from build123d import *

# Parameters (mm, degrees)
F0_W     = 10
F0_H     = 10
F1_DEPTH = 3.75


with BuildPart() as f1:
    # F0 (on Front) → F1 (new body, symmetric)
    with BuildSketch(Plane.XZ):
        with BuildLine():
            Line((13.240477, 26.920062), (-1.299121, 22.463483))
            Line((-1.299121, 22.463483), (0.005236, 30))
            ThreePointArc((0.005236, 30), (-0.994655, 29.983506), (-1.993441, 29.933697))
            Line((-1.993441, 29.933697), (-12.356813, 18.804386))
            Line((-12.356813, 18.804386), (-14.995465, 25.98338))
            ThreePointArc((-14.995465, 25.98338), (-15.85315, 25.469151), (-16.693219, 24.926621))
            Line((-16.693219, 24.926621), (-20.103507, 10.10667))
            Line((-20.103507, 10.10667), (-25.978144, 15.004534))
            ThreePointArc((-25.978144, 15.004534), (-26.463806, 14.130356), (-26.920062, 13.240477))
            Line((-26.920062, 13.240477), (-22.463483, -1.299121))
            Line((-22.463483, -1.299121), (-30, 0.005236))
            ThreePointArc((-30, 0.005236), (-29.983506, -0.994655), (-29.933697, -1.993441))
            Line((-29.933697, -1.993441), (-18.804386, -12.356813))
            Line((-18.804386, -12.356813), (-25.98338, -14.995465))
            ThreePointArc((-25.98338, -14.995465), (-25.469151, -15.85315), (-24.926621, -16.693219))
            Line((-24.926621, -16.693219), (-10.10667, -20.103507))
            Line((-10.10667, -20.103507), (-15.004534, -25.978144))
            ThreePointArc((-15.004534, -25.978144), (-14.130356, -26.463806), (-13.240477, -26.920062))
            Line((-13.240477, -26.920062), (1.299121, -22.463483))
            Line((1.299121, -22.463483), (-0.005236, -30))
            ThreePointArc((-0.005236, -30), (0.994655, -29.983506), (1.993441, -29.933697))
            Line((1.993441, -29.933697), (12.356813, -18.804386))
            Line((12.356813, -18.804386), (14.995465, -25.98338))
            ThreePointArc((14.995465, -25.98338), (15.85315, -25.469151), (16.693219, -24.926621))
            Line((16.693219, -24.926621), (20.103507, -10.10667))
            Line((20.103507, -10.10667), (25.978144, -15.004534))
            ThreePointArc((25.978144, -15.004534), (26.463806, -14.130356), (26.920062, -13.240477))
            Line((26.920062, -13.240477), (22.463483, 1.299121))
            Line((22.463483, 1.299121), (30, -0.005236))
            ThreePointArc((30, -0.005236), (29.983506, 0.994655), (29.933697, 1.993441))
            Line((29.933697, 1.993441), (18.804386, 12.356813))
            Line((18.804386, 12.356813), (25.98338, 14.995465))
            ThreePointArc((25.98338, 14.995465), (25.469151, 15.85315), (24.926621, 16.693219))
            Line((24.926621, 16.693219), (10.10667, 20.103507))
            Line((10.10667, 20.103507), (15.004534, 25.978144))
            ThreePointArc((15.004534, 25.978144), (14.130356, 26.463806), (13.240477, 26.920062))
        make_face()
        Rectangle(F0_W, F0_H, mode=Mode.SUBTRACT)
    extrude(amount=F1_DEPTH, both=True)


solid = f1.part
Part model, mm, in its own coordinate system. A direction names the side the tool comes from. Coordinates: 2 decimals unless noted, no trailing zeros. Order: outer loops, then holes, each group sorted by start corner. A loop starts at its lowest first (then second) coordinate and runs counter-clockwise, first axis right, second up.
(1) Slice it at D-D, the plane x = -9. Write the cut outline in (y, z).
Check sheet entries:
outline: (-3.75, -25.62) - (3.75, -25.62) - (3.75, 22.41) - (-3.75, 22.41) - close
(2) Slice it at A-A, the plane z = -4. Write the cut outline in (x, y).
Check sheet entries:
outline: (-27.78, -3.75) - (-5, -3.75) - (-5, 3.75) - (-27.78, 3.75) - close; (5, -3.75) - (24.09, -3.75) - (24.09, 3.75) - (5, 3.75) - close
(3) Pin check, flat tips, straight feed: pin 1 Ø4 at (x, y) = (-16.5, 2.5) entering from +Z; pin 2 Ø2 at (x, y) = (-5.5, -1.5) entering from -Z; pin 3 Ø1 at (y, z) = (-1, -1.5) entering from +X. Stop position of each tip, or through.
Check sheet entries:
pin 1: stops at z = 25.98
pin 2: stops at z = -24.85
pin 3: stops at x = 23.47
(4) Pull direction Z, two halves, no side cores. Call faces 5 (the face through (6, 3.75, 0)), 6 (the face through (0.656, -0.053, -26.179)), 7 (the face through (7.1, -0.05, -24.45)): pulls with the +Z half, pulls with the -Z half, needs draft (parallel to the pull), parting line crosses it, or undercut.
Check sheet entries:
face 5: needs draft
face 6: undercut
face 7: pulls with the -Z half
(5) Tool access for faces 1 (the face through (12.52, -0.05, 23)), 2 (the face through (-22.344, -0.053, -13.658)), 3 (the face through (23, -0.05, -12.52)), 4 (the face through (-23, -0.05, 12.52)): list every direction of +Z, -Z, +X, -X, +Y, -Y with a clear straight run to the whole face (end or side of a thin tool).
Check sheet entries:
face 1: +X, +Y, -Y
face 2: -X, +Y, -Y
face 3: -Z, +Y, -Y
face 4: +Z, +Y, -Y
(6) Slice it at C-C, the plane z = 7. Write the cut outline in (x, y).
Check sheet entries:
outline: (-25.01, -3.75) - (24.56, -3.75) - (24.56, 3.75) - (-25.01, 3.75) - close
(7) Probe L1, parallel to X at y = 0.5, z = -3; L2, parallel to Z at x = -11.5, y = 0.25; L3, parallel to Z at x = 12, y = 1.5. List the from-to ranges inside material, lowest first.
Check sheet entries:
L1: x = -28.85 to -5, 5 to 23.78
L2: z = -26.39 to -21.77, -19.78 to 19.72
L3: z = -19.19 to 19.67, 22.37 to 26.54
(8) Slice it at B-B, the plane x = 3.5. Write the cut outline in (y, z), and give its area (3 significant figures).
Check sheet entries:
outline: (-3.75, -28.32) - (3.75, -28.32) - (3.75, -5) - (-3.75, -5) - close; (-3.75, 5) - (3.75, 5) - (3.75, 23.93) - (-3.75, 23.93) - close
area: 317 mm2
